The model under review builds one solid part; all positions refer to its coordinate system, in mm. Face numbers are marked on the shaded views. Coordinates: 2 decimals unless noted, no trailing zeros. Order: outer loops, then holes, each group sorted by start corner. A loop starts at its lowest first (then second) coordinate and runs counter-clockwise, first axis right, second up. Notation, with made-up numbers: (28, -14.75) -> (70, -14.75) arc R10 cw to (70, -1.75) -> close; hole circle Ø4 at (73.25, 72.5). An arc over 180 degrees is marked (long way). Put each result on its own line as item: value.
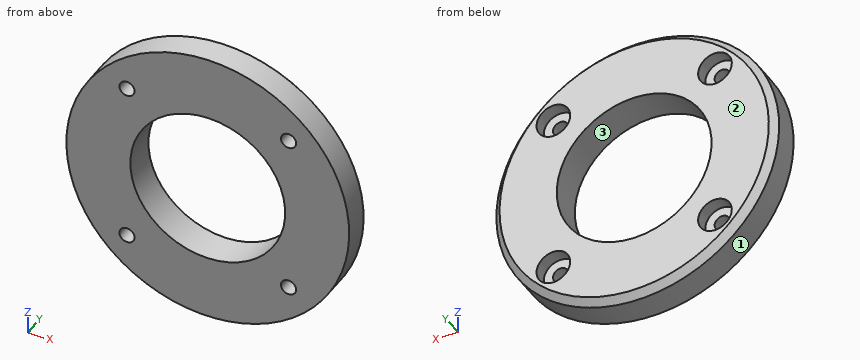
from build123d import *

# Parameters (mm, degrees)
SKETCH1_R                               = 42
SKETCH1_R_2                             = 23
EXTRUDE1_DEPTH                          = 10
CBORE_FOR_M4_HEX_HEAD_BOLT1_D           = 4.5
CBORE_FOR_M4_HEX_HEAD_BOLT1_DEPTH       = 19.75
CBORE_FOR_M4_HEX_HEAD_BOLT1_CBORE_D     = 10
CBORE_FOR_M4_HEX_HEAD_BOLT1_CBORE_DEPTH = 4
CBORE_FOR_M4_HEX_HEAD_BOLT1_TIP         = 1.351936393
CHAMFER2_SIZE                           = 2


with BuildPart() as part:
    # Sketch1 → Extrude1 (new body)
    with BuildSketch(Plane(origin=(0, 0, 0), x_dir=(1, 0, 0), z_dir=(0, 1, 0))):
        with Locations(Location((0, 0, 0), (0, 0, 270))):
            Circle(SKETCH1_R)
        with Locations(Location((0, 0, 0), (0, 0, 270))):
            Circle(SKETCH1_R_2, mode=Mode.SUBTRACT)
    extrude(amount=EXTRUDE1_DEPTH)

    # CBORE for M4 Hex Head Bolt1
    with Locations(Plane(origin=(-24, 10, -24), x_dir=(0, 0, 1), z_dir=(0, 1, 0))):
        with Locations((0, 0), (0, 48), (48, 48), (48, 0)):
            CounterBoreHole(CBORE_FOR_M4_HEX_HEAD_BOLT1_D / 2, CBORE_FOR_M4_HEX_HEAD_BOLT1_CBORE_D / 2, CBORE_FOR_M4_HEX_HEAD_BOLT1_CBORE_DEPTH, depth=CBORE_FOR_M4_HEX_HEAD_BOLT1_DEPTH)
            with Locations((0, 0, -(CBORE_FOR_M4_HEX_HEAD_BOLT1_DEPTH + CBORE_FOR_M4_HEX_HEAD_BOLT1_TIP / 2))):  # 118° drill point
                Cone(0, CBORE_FOR_M4_HEX_HEAD_BOLT1_D / 2, CBORE_FOR_M4_HEX_HEAD_BOLT1_TIP, mode=Mode.SUBTRACT)

    # Chamfer2
    chamfer2_edges = [part.edges().sort_by_distance(p)[0] for p in [
        (0, 10, -42),
    ]]
    chamfer(chamfer2_edges, length=CHAMFER2_SIZE)


solid = part.part
Item 1: Consider section B-B on x = 0. Write out the cut boundary in (y, z), and give its area (3 significant figures).
Answers below:
outline: (0, -42) -> (8, -42) -> (10, -40) -> (10, -23) -> (0, -23) -> close; (0, 23) -> (10, 23) -> (10, 40) -> (8, 42) -> (0, 42) -> close
area: 376 mm^2
Item 2: Consider section A-A on z = 0. Write out the cut boundary in (x, y).
Answers below:
outline: (-42, 0) -> (-23, 0) -> (-23, 10) -> (-40, 10) -> (-42, 8) -> close; (23, 0) -> (42, 0) -> (42, 8) -> (40, 10) -> (23, 10) -> close
Item 3: Consider section D-D on z = -24. Count the separate pieces of the cut face and the enclosed holes in it, and give its area (3 significant figures).
Answers below:
separate pieces: 3
enclosed holes: 0
area: 550 mm^2
Item 4: For pin 1 Ø3 at (x, y) = (19.5, 4) entering from -Z; pin 2 Ø8 at (x, z) = (22, -21.5) entering from +Y; pin 3 Ø4 at (x, y) = (18.5, 2.5) entering from -Z; pin 4 Ø3.5 at (x, z) = (-24, -24) entering from +Y, all flat-tipped, find the tip position at first contact; note any pin that passes through.
Answers below:
pin 1: z = -37.95
pin 2: y = 10
pin 3: z = -38.62
pin 4: through
Item 5: Mouldability with a two-part tool opening along Z and no side actions: class the marked faces 1, 2 and 3 as +Z half, -Z half, draft (parallel to the pull), parting line (faces both ways), or undercut.
Answers below:
face 1: parting line
face 2: draft
face 3: undercut
Item 6: For line 1 (X direction, y = 9.05, z = 24); line 2 (X direction, y = 7, z = 20); line 3 (Z direction, x = 0.5, y = 3.25), list the stretches that pass through material, from the lowest coordinate up. Write a range as from..to.
Answers below:
line 1: -33.18..-29, -19..19, 29..33.18
line 2: -36.93..-27, -21..-11.36, 11.36..21, 27..36.93
line 3: -42..-22.99, 22.99..42
Item 7: Consider section C-C on y = 3.5. Write out the cut boundary in (x, z), and give its area (3 significant figures).
Answers below:
outline: circle Ø84 at (0, 0); hole circle Ø4.5 at (-24, -24); hole circle Ø4.5 at (-24, 24); hole circle Ø46 at (0, 0); hole circle Ø4.5 at (24, -24); hole circle Ø4.5 at (24, 24)
area: 3,820 mm^2
